The drawing under review shows one solid part. Ordinate dimensions are in mm from its lowest x, y, z. Give positions to 0.01 mm unless a question says otherwise; leave off trailing zeros. Loops run counter-clockwise (first coordinate to the right, second up) from the corner with the lowest first, then second, coordinate; pieces in that order, holes last. Notation, with made-up numbers: (11, 53.5) - (63, 53.5) arc R4 cw to (63, 59.5) - close; hole circle Ø6 at (47.5, -6.75). An arc over 180 degrees is marked (long way). Return JSON: item names as keys, results as strings. Group by question number.
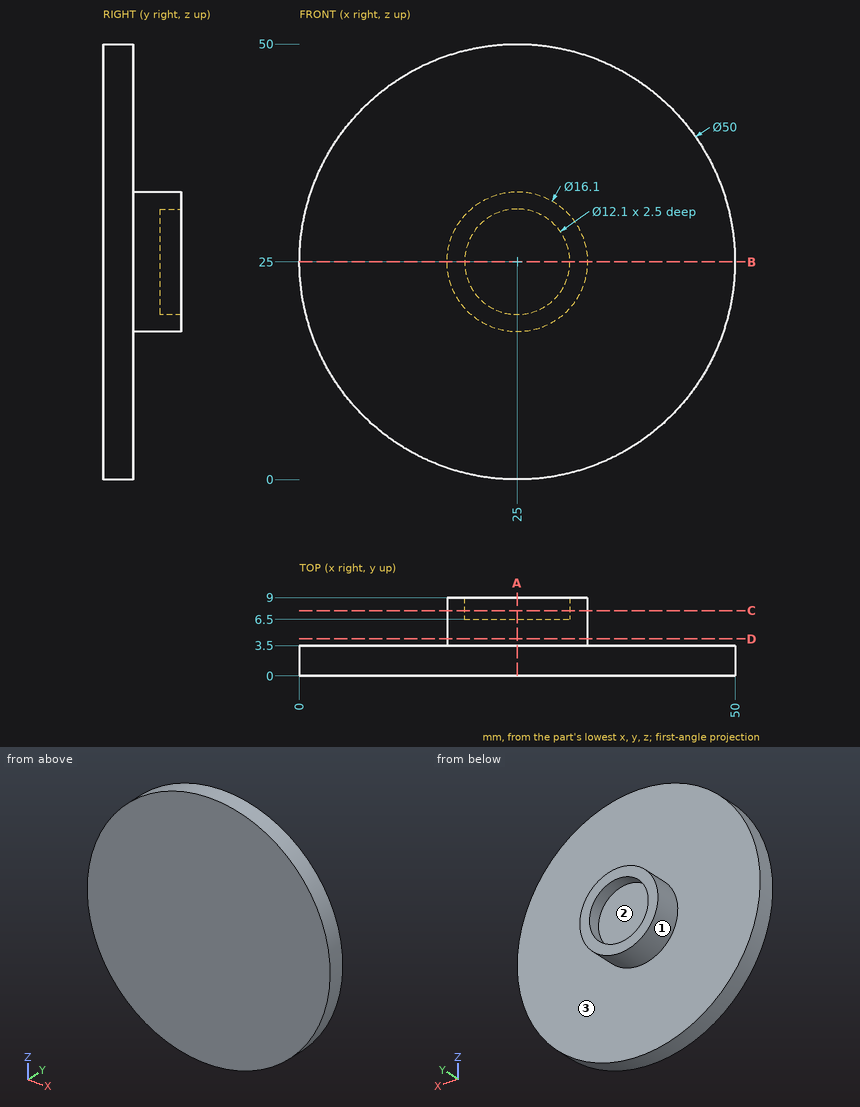
1) We need section C-C, the plane y = 7.5. Write out the cut boundary in (x, z), plus the area to 3 significant figures.
2) We need section A-A, the plane x = 25. Write out the cut boundary in (y, z), plus the area to 3 significant figures.
3) To check wall thickness, follow line 1 (X direction, y = 8.55, z = 25); line 2 (Y direction, x = 39.5, z = 33); line 3 (Y direction, x = 28, z = 21.5). State the ranges of each line that lie inside material, in increasing order.
4) Draft analysis for pull direction X (two halves, no side actions). For the marked faces 1, 2 and 3, state which applies: +X half, -X half, draft (parallel to the pull), parting line (faces both ways), or undercut.
5) For pin 1 Ø4 at (x, z) = (30.5, 27) entering from +Y; pin 2 Ø6 at (x, z) = (27, 23) entering from +Y; pin 3 Ø5 at (x, y) = (34, 7) entering from +Z, all flat-tipped, find the tip position at first contact; note any pin that passes through.
6) We need section B-B, the plane z = 25. Write out the cut boundary in (x, y), plus the area to 3 significant figures.
7) We need section D-D, the plane y = 4.25. Write out the cut boundary in (x, z).
Findings:
{
 "1": {"outline": "circle Ø16.1 at (25, 25); hole circle Ø12.1 at (25, 25)", "area": "88.6 mm^2"},
 "2": {"outline": "(0, 0) - (3.5, 0) - (3.5, 16.95) - (9, 16.95) - (9, 18.95) - (6.5, 18.95) - (6.5, 31.05) - (9, 31.05) - (9, 33.05) - (3.5, 33.05) - (3.5, 50) - (0, 50) - close", "area": "233 mm^2"},
 "3": {"line 1": "x = 16.95 to 18.95, 31.05 to 33.05", "line 2": "y = 0 to 3.5", "line 3": "y = 0 to 6.5"},
 "4": {"face 1": "parting line", "face 2": "undercut", "face 3": "draft"},
 "5": {"pin 1": "stops at y = 9", "pin 2": "stops at y = 6.5", "pin 3": "stops at z = 29.75"},
 "6": {"outline": "(0, 0) - (50, 0) - (50, 3.5) - (33.05, 3.5) - (33.05, 9) - (31.05, 9) - (31.05, 6.5) - (18.95, 6.5) - (18.95, 9) - (16.95, 9) - (16.95, 3.5) - (0, 3.5) - close", "area": "233 mm^2"},
 "7": {"outline": "circle Ø16.1 at (25, 25)"}
}
